from build123d import *

# Parameters (mm, degrees)
SKETCH_1_W          = 73
SKETCH_1_H          = 47
SKETCH_1_R          = 1
EXTRUDE_1_DEPTH     = 10
FILLET_1_R          = 3
SKETCH_3_R          = 2
CUT_EXTRUDE_1_DEPTH = 1
SKETCH_2_R          = 2.5
EXTRUDE_2_DEPTH     = 8.5
EXTRUDE_START       = 9
SKETCH_5_R          = 2.5
EXTRUDE_3_DEPTH     = 9
SKETCH_6_W          = 8
SKETCH_6_H          = 4
LAN_DEPTH           = 2
SKETCH_7_W          = 11
SKETCH_7_H          = 4
COM_DEPTH           = 2
SKETCH_8_W          = 10
SKETCH_8_H          = 5.2
XT30_DEPTH          = 7


with BuildPart() as part:
    # 草图1 → 凸台-拉伸1 (new body)
    with BuildSketch(Plane(origin=(0, 0, 0), x_dir=(1, 0, 0), z_dir=(0, 1, 0))):
        with Locations((36.5, 23.5)):
            Rectangle(SKETCH_1_W, SKETCH_1_H)
        with Locations(Location((4, 3.5, 0), (0, 0, 270))):
            Circle(SKETCH_1_R, mode=Mode.SUBTRACT)
        with Locations(Location((4, 43.5, 0), (0, 0, 90))):
            Circle(SKETCH_1_R, mode=Mode.SUBTRACT)
        with Locations(Location((69, 3.5, 0), (0, 0, 90))):
            Circle(SKETCH_1_R, mode=Mode.SUBTRACT)
        with Locations(Location((69, 43.5, 0), (0, 0, 270))):
            Circle(SKETCH_1_R, mode=Mode.SUBTRACT)
    extrude(amount=EXTRUDE_1_DEPTH)

    # 圆角1
    fillet_1_edges = [part.edges().sort_by_distance(p)[0] for p in [
        (0, 5, -47),
        (73, 5, -47),
        (73, 5, 0),
        (0, 5, 0),
    ]]
    fillet(fillet_1_edges, radius=FILLET_1_R)

    # 草图3 → 切除-拉伸1 (cut)
    with BuildSketch(Plane.XZ):
        with Locations(Location((4, -43.5, 0), (0, 0, 270))):
            Circle(SKETCH_3_R)
        with Locations(Location((4, -3.5, 0), (0, 0, 270))):
            Circle(SKETCH_3_R)
        with Locations(Location((69, -3.5, 0), (0, 0, 270))):
            Circle(SKETCH_3_R)
        with Locations(Location((69, -43.5, 0), (0, 0, 270))):
            Circle(SKETCH_3_R)
    extrude(amount=-CUT_EXTRUDE_1_DEPTH, mode=Mode.SUBTRACT)

    # 草图2 → 凸台-拉伸2 (add)
    with BuildSketch(Plane(origin=(0, 0, -47), x_dir=(-1, 0, 0), z_dir=(0, 0, -1))):
        with Locations(Location((-12, 5, 0), (0, 0, 180))):
            Circle(SKETCH_2_R)
    extrude(amount=EXTRUDE_2_DEPTH)

    # 草图5 → 凸台-拉伸3 (add)
    with BuildSketch(Plane.XY.offset(EXTRUDE_START)):
        with Locations((12, 5)):
            Circle(SKETCH_5_R)
    extrude(amount=-EXTRUDE_3_DEPTH)

    # 草图6 → LAN口预留 (add)
    with BuildSketch(Plane.XY):
        with Locations((42, 4)):
            Rectangle(SKETCH_6_W, SKETCH_6_H)
    extrude(amount=LAN_DEPTH)

    # 草图7 → COM口预留 (add)
    with BuildSketch(Plane(origin=(0, 0, -47), x_dir=(-1, 0, 0), z_dir=(0, 0, -1))):
        with Locations((-53.5, 4)):
            Rectangle(SKETCH_7_W, SKETCH_7_H)
    extrude(amount=COM_DEPTH)

    # 草图8 → XT30预留 (add)
    with BuildSketch(Plane(origin=(73, 0, 0), x_dir=(0, 0, -1), z_dir=(1, 0, 0))):
        with Locations((14, 3.4)):
            Rectangle(SKETCH_8_W, SKETCH_8_H)
    extrude(amount=XT30_DEPTH)


solid = part.part
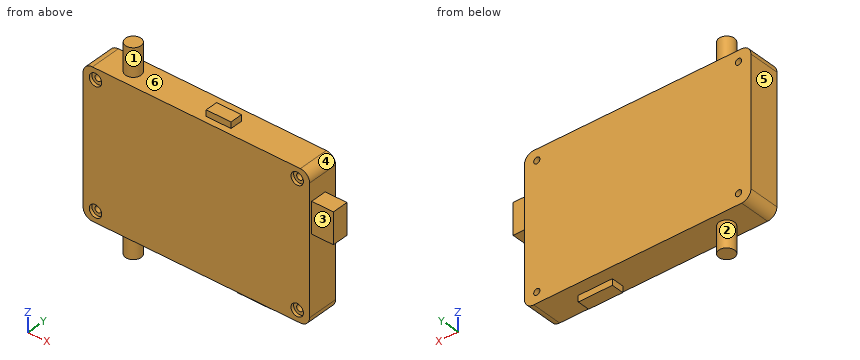
Read the model definition and answer for the solid it produces. Units are mm, in the model's axes. Face numbers are marked on the shaded views. A direction names the side the tool comes from. Coordinates: 2 decimals unless noted, no trailing zeros. Loops run counter-clockwise (first coordinate to the right, second up) from the corner with the lowest first, then second, coordinate; pieces in that order, holes last. Notation, with made-up numbers: (46, 32.5) -> (105, 32.5) arc R32 cw to (105, 70.5) -> close; hole circle Ø5 at (29, 2). An arc over 180 degrees is marked (long way). Write item = value, one per line. Start each with the question number.
1) The mould has two halves that part along X. Classify the marked faces 4, 5 and 6: pulls with the +X half, pulls with the -X half, needs draft (parallel to the pull), parting line crosses it, or undercut.
2) Find the intervals of material crossed by L1, parallel to Z at x = 69, y = 7; L2, parallel to X at y = 0.7, z = -3.5; L3, parallel to X at y = 6.5, z = -3.5, in increasing order. Write a range as from..to.
3) The part is cut by section D-D, the plane z = -21. Determine the outline of the cut face in (x, y), plus the area to 3 significant figures.
4) The part is cut by section B-B, the plane y = 5. State how many separate pieces and enclosed holes the cut face has, plus the area to 3 significant figures.
5) Given P1, Ø1, axis at x = 21, y = 6, coming from the +Z side; P2, Ø4, axis at x = 62.5, y = 6.5, coming from the -Z side; P3, Ø4, axis at x = 78, y = 4.5, coming from the +Z side; P4, Ø1.8, axis at x = 4, z = -43.5, coming from the -Y side, each flat-ended and moving along its own axis, determine where each tip first touches the part or whether it passes through.
6) For the marked faces 1, 2 and 3, determine the directions among +Z, -Z, +X, -X, +Y, -Y from which every point of the face is accessible in a straight line to the end or side of a thin tool.
7) The part is cut by section A-A, the plane x = 4. Determine the outline of the cut face in (y, z), plus the area to 3 significant figures.
8) The part is cut by section C-C, the plane x = 12. Determine the outline of the cut face in (y, z), plus the area to 4 significant figures.
Result:
q1.face_4 = pulls with the +X half
q1.face_5 = pulls with the -X half
q1.face_6 = undercut
q2.L1 = -47..-44.5, -42.5..-4.5, -2.5..0
q2.L2 = 0..2, 6..67, 71..73
q2.L3 = 0..3, 5..68, 70..73
q3.outline = (0, 0) -> (73, 0) -> (73, 10) -> (0, 10) -> close
q3.area = 730 mm²
q4.separate_pieces = 1
q4.enclosed_holes = 4
q4.area = 3,610 mm²
q5.P1 = 0
q5.P2 = -47
q5.P3 = -9
q5.P4 = through
q6.face_1 = +Z
q6.face_2 = -Z
q6.face_3 = +Z, -Z, +X, -Y
q7.outline = (0, -47) -> (10, -47) -> (10, -44.5) -> (1, -44.5) -> (1, -45.5) -> (0, -45.5) -> close; (0, -41.5) -> (1, -41.5) -> (1, -42.5) -> (10, -42.5) -> (10, -4.5) -> (1, -4.5) -> (1, -5.5) -> (0, -5.5) -> close; (0, -1.5) -> (1, -1.5) -> (1, -2.5) -> (10, -2.5) -> (10, 0) -> (0, 0) -> close
q7.area = 426 mm²
q8.outline = (0, -47) -> (2.5, -47) -> (2.5, -55.5) -> (7.5, -55.5) -> (7.5, -47) -> (10, -47) -> (10, 0) -> (7.5, 0) -> (7.5, 9) -> (2.5, 9) -> (2.5, 0) -> (0, 0) -> close
q8.area = 557.5 mm²
